```python
from build123d import *

# Parameters (mm, degrees)
F0_W     = 5
F0_H     = 5
F1_DEPTH = 3
F2_DEPTH = 4


with BuildPart() as f1:
    # F0 (on Right) → F1 (new body)
    with BuildSketch(Plane.YZ):
        with Locations((41.605493, 33.802644)):
            Rectangle(F0_W, F0_H)
    extrude(amount=F1_DEPTH)

    # F0 (on Right) → F2 (join)
    with BuildSketch(Plane.YZ):
        Polygon((45.93562, 41.302644), (37.275366, 41.302644), (32.945239, 33.802644), (37.275366, 26.302644), (45.93562, 26.302644), (50.265747, 33.802644), align=None)
        with Locations((41.605493, 33.802644)):
            Rectangle(F0_W, F0_H, mode=Mode.SUBTRACT)
        with Locations((41.605493, 33.802644)):
            Rectangle(F0_W, F0_H)
    extrude(amount=-F2_DEPTH)


solid = f1.part
```
Source: CAD feature listing. Evaluate the final solid. Frame: model axes, mm. A direction names the side the tool comes from. Give positions to 0.01 mm unless a question says otherwise; leave off trailing zeros. Loops run counter-clockwise (first coordinate to the right, second up) from the corner with the lowest first, then second, coordinate; pieces in that order, holes last. Notation, with made-up numbers: (63.5, 56.25) - (106.5, 56.25) arc R10 cw to (106.5, 63.25) - close; hole circle Ø3 at (0.5, 89.25). An arc over 180 degrees is marked (long way). Use CSV: the item, a comma, the result in double quotes. Start each with the question number.
1. Reachability of faces 1 (the flat face through (1, 42, 31.303)), 2 (the flat face through (-2, 42, 41.303)), 3 (the flat face through (1, 42, 36.303)), 4 (the flat face through (1, 44.105, 34)), 5 (the flat face through (1, 39.105, 34)) from +Z, -Z, +X, -X, +Y, -Y: full face, straight path, thin tool, end or side. Return the list, or none.
2. Section A-A (y = 43.75). Output: boundary loops of the cut face in (x, z).
3. Ray query, L1, parallel to X at y = 35.25, z = 33; L2, parallel to Y at x = 0.25, z = 34; L3, parallel to Z at x = 2.75, y = 41.5. Return the intervals inside material, ascending.
4. Pin query (flat end, axial travel): pin 1 (3 mm diameter, centred on x = -2, z = 29.5, fed in from -Y); pin 2 (2.5 mm diameter, centred on x = 1.5, y = 43, fed in from +Z); pin 3 (1.5 mm diameter, centred on x = 1.5, z = 35, fed in from +Y). Return the tip coordinate at first contact, or that it passes through.
5. Section C-C (z = 36). Output: boundary loops of the cut face in (x, y).
6. Section D-D (x = 2.5). Output: boundary loops of the cut face in (y, z), then the cut area to 3 significant figures.
7. Section B-B (x = -1.75). Output: boundary loops of the cut face in (y, z), then the cut area to 3 significant figures.
Response:
1,face 1,"-Z, +X, +Y, -Y"
1,face 2,"+Z, +X, -X, +Y, -Y"
1,face 3,"+Z, +X, +Y, -Y"
1,face 4,"+Z, -Z, +X, +Y"
1,face 5,"+Z, -Z, +X, -Y"
2,outline,"(-4, 26.3) - (0, 26.3) - (0, 31.3) - (3, 31.3) - (3, 36.3) - (0, 36.3) - (0, 41.3) - (-4, 41.3) - close"
3,L1,"-4 to 0"
3,L2,"39.11 to 44.11"
3,L3,"31.3 to 36.3"
4,pin 1,"y = 34.56"
4,pin 2,"z = 36.3"
4,pin 3,"y = 44.11"
5,outline,"(-4, 34.21) - (0, 34.21) - (0, 39.11) - (3, 39.11) - (3, 44.11) - (0, 44.11) - (0, 49) - (-4, 49) - close"
6,outline,"(39.11, 31.3) - (44.11, 31.3) - (44.11, 36.3) - (39.11, 36.3) - close"
6,area,"25.0 mm²"
7,outline,"(32.95, 33.8) - (37.28, 26.3) - (45.94, 26.3) - (50.27, 33.8) - (45.94, 41.3) - (37.28, 41.3) - close"
7,area,"195 mm²"
